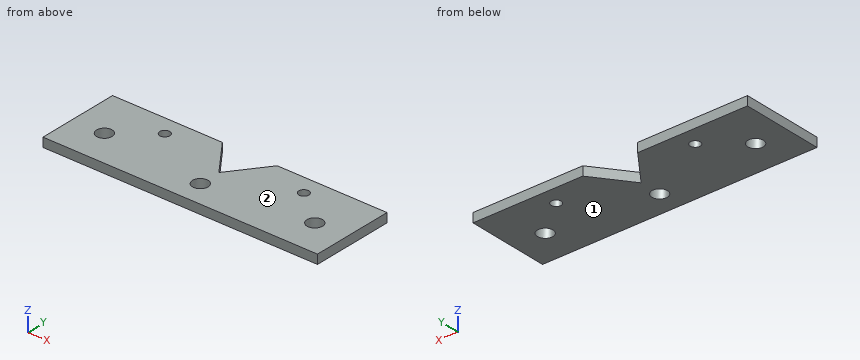
from build123d import *

# Parameters (mm, degrees)
SKETCH1_R           = 4.25
SKETCH1_R_2         = 2.75
BOSS_EXTRUDE1_DEPTH = 5


with BuildPart() as part:
    # Sketch1 → Boss-Extrude1 (new body)
    with BuildSketch(Plane.XY):
        Polygon((-127.499192618, 23.526116329), (-127.499192618, 68.526116329), (-67.499192618, 68.526116329), (-52.499192618, 48.526116329), (-37.499192618, 68.526116329), (22.500807382, 68.526116329), (22.500807382, 23.526116329), align=None)
        with Locations((-109.999192618, 42.526116329)):
            Circle(SKETCH1_R, mode=Mode.SUBTRACT)
        with Locations((5.000807382, 42.526116329)):
            Circle(SKETCH1_R, mode=Mode.SUBTRACT)
        with Locations((-52.499192618, 36.526116329)):
            Circle(SKETCH1_R, mode=Mode.SUBTRACT)
        with Locations((-90.499192618, 58.526116329)):
            Circle(SKETCH1_R_2, mode=Mode.SUBTRACT)
        with Locations((-14.499192618, 58.526116329)):
            Circle(SKETCH1_R_2, mode=Mode.SUBTRACT)
    extrude(amount=BOSS_EXTRUDE1_DEPTH)


solid = part.part
Verification items for the finished model (mm, model axes). Face numbers are marked on the shaded views. Give positions to 0.01 mm unless a question says otherwise; leave off trailing zeros. Write each loop counter-clockwise with the first axis right and the second up, starting at its lowest first coordinate (ties: lowest second). Pieces come first, ordered by that corner, then holes. Notation, with made-up numbers: (66.5, 89) - (77.5, 89) arc R23 cw to (77.5, 108) - close; hole circle Ø6 at (84, -9.75). An arc over 180 degrees is marked (long way). Answer as CSV lines item,"result". Start each with the question number.
1. Draft check along Z on the marked faces 1 and 2. Enter one of: pulls with the +Z half, pulls with the -Z half, needs draft (parallel to the pull), parting line crosses it, or undercut.
2. Thickness scan on line 1 (X direction, y = 43.5, z = 4); line 2 (X direction, y = 59.5, z = 0.55); line 3 (X direction, y = 60.5, z = 4.35). Record the ranges inside material, lowest first.
3. Sectioned sample at B-B (z = 2.75). Record the boundary of the cut face in (x, y), then the cut area to 3 significant figures.
4. Sectioned sample at A-A (x = -108.5). Record the boundary of the cut face in (y, z).
5. Sectioned sample at C-C (x = -15). Record the boundary of the cut face in (y, z).
6. Sectioned sample at D-D (x = -42). Record the boundary of the cut face in (y, z).
Derived:
1,face 1,"pulls with the -Z half"
1,face 2,"pulls with the +Z half"
2,line 1,"-127.5 to -114.14, -105.86 to 0.86, 9.14 to 22.5"
2,line 2,"-127.5 to -93.07, -87.93 to -60.73, -44.27 to -17.07, -11.93 to 22.5"
2,line 3,"-127.5 to -92.41, -88.58 to -61.48, -43.52 to -16.41, -12.58 to 22.5"
3,outline,"(-127.5, 23.53) - (22.5, 23.53) - (22.5, 68.53) - (-37.5, 68.53) - (-52.5, 48.53) - (-67.5, 68.53) - (-127.5, 68.53) - close; hole circle Ø8.5 at (-110, 42.53); hole circle Ø5.5 at (-90.5, 58.53); hole circle Ø8.5 at (-52.5, 36.53); hole circle Ø5.5 at (-14.5, 58.53); hole circle Ø8.5 at (5, 42.53)"
3,area,"6,230 mm²"
4,outline,"(23.53, 0) - (38.55, 0) - (38.55, 5) - (23.53, 5) - close; (46.5, 0) - (68.53, 0) - (68.53, 5) - (46.5, 5) - close"
5,outline,"(23.53, 0) - (55.82, 0) - (55.82, 5) - (23.53, 5) - close; (61.23, 0) - (68.53, 0) - (68.53, 5) - (61.23, 5) - close"
6,outline,"(23.53, 0) - (62.53, 0) - (62.53, 5) - (23.53, 5) - close"
